Study the drawing (mm; zero at the part's minimum x, y, z) and answer. Round coordinates to 2 decimals unless told otherwise and drop trailing zeros. Write each loop counter-clockwise with the first axis right and the second up, starting at its lowest first coordinate (ties: lowest second). Pieces come first, ordered by that corner, then holes. Notation, with made-up numbers: (85.5, -14.75) - (97.5, -14.75) arc R18 cw to (97.5, -5.75) - close; hole circle Ø6 at (32.5, 5). An arc over 180 degrees is marked (long way). Use one line per item in the form item = value. Start each with the question number.
1) The part is cut by section B-B, the plane x = 2.5. Give the vertices of the cut face in (y, z), plus the area to 3 significant figures.
2) Consider line 1 along Z through (x, y) = (3, 1.7); line 2 along X through (y, z) = (0.65, 66.5); line 3 along X through (y, z) = (2.5, 68.5). Determine where each line is inside the solid, lowest interval first. Write a range as from..to.
3) The part is cut by section A-A, the plane y = 1.35. Give the vertices of the cut face in (x, z), plus the area to 3 significant figures.
4) The part is cut by section C-C, the plane z = 71.5. Give the vertices of the cut face in (x, y).
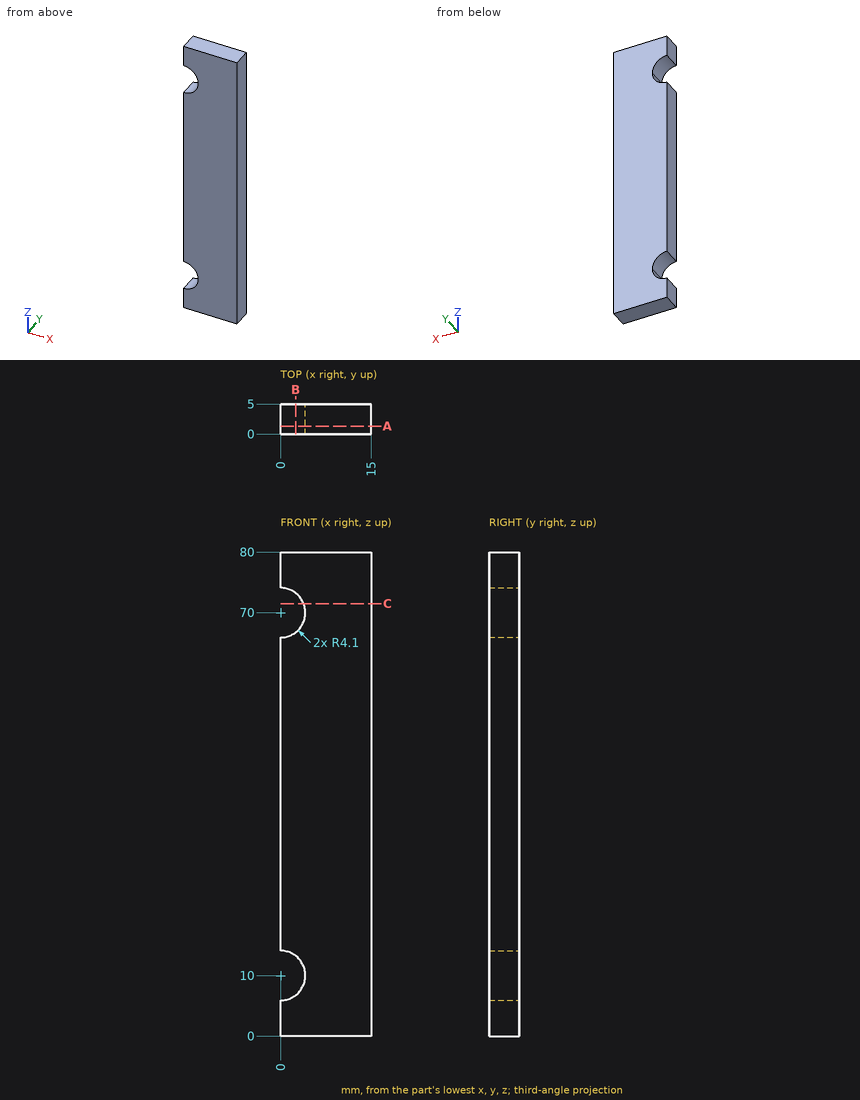
Geometry results:
q1.outline = (0, 0) - (5, 0) - (5, 6.75) - (0, 6.75) - close; (0, 13.25) - (5, 13.25) - (5, 66.75) - (0, 66.75) - close; (0, 73.25) - (5, 73.25) - (5, 80) - (0, 80) - close
q1.area = 335 mm2
q2.line_1 = 0..7.21, 12.79..67.21, 72.79..80
q2.line_2 = 2.14..15
q2.line_3 = 3.82..15
q3.outline = (0, 0) - (15, 0) - (15, 80) - (0, 80) - (0, 74.1) arc R4.1 cw to (0, 65.9) - (0, 14.1) arc R4.1 cw to (0, 5.9) - close
q3.area = 1,150 mm2
q4.outline = (3.82, 0) - (15, 0) - (15, 5) - (3.82, 5) - close
